Geometry: final body of the model. Coordinates: model frame, mm. Face numbers are marked on the shaded views. A direction names the side the tool comes from. Coordinates: 2 decimals unless noted, no trailing zeros. Order: outer loops, then holes, each group sorted by start corner. A loop starts at its lowest first (then second) coordinate and runs counter-clockwise, first axis right, second up. Notation, with made-up numbers: (81, -4.5) -> (98, -4.5) arc R11 ccw to (98, 1.5) -> close; hole circle Ø11 at (30.5, 37.5). An arc over 180 degrees is marked (long way). Answer in a Markdown table with one row per item. Add a question column.
1) Set-up query: the marked faces 1 and 2. Return all of +Z, -Z, +X, -X, +Y, -Y with unobstructed straight access to the full face (end or side cutting, diameter ignored); none if empty.
2) Contact query for flat-ended pins moving along their axis: P1, Ø1.8, axis at x = -3, z = 17, coming from the +Y side; P2, Ø6, axis at x = -5, y = -48.5, coming from the +Z side; P3, Ø5.5, axis at y = -10.5, z = 29, coming from the -X side. Output: stop coordinate, or through.
3) Ray query, line 1 (Y direction, x = -15.5, z = 19.5); line 2 (X direction, y = -33, z = 18.5); line 3 (X direction, y = -45.5, z = 18.25). Return the intervals inside material, ascending. Write a range as from..to.
4) Section query B-B on z = 20. Return the cut outline in (x, y), then the cut area to 3 significant figures.
5) Section query C-C on y = -20. Return the cut outline in (x, z), then the cut area to 3 significant figures.
```python
from build123d import *

# Parameters (mm, degrees)
F1_DEPTH = 50
F2_W     = 43.9973853057
F2_H     = 6
F3_DEPTH = 125


# Not quite as in the source:
# - ends of sketch curves that miss each other by under 0.0002 mm in the source are joined
# - a feature names something its author has since deleted; it is built from what else it names


with BuildPart() as f1:
    # F0 (on Top) → F1 (new body, symmetric)
    with BuildSketch(Plane.XY):
        Polygon((15.8618143265, -2.6014313847), (15.8618143265, -13.6014313847), (50.9007196128, -13.6014313847), (50.8959237908, -2.6014324301), align=None)
        with BuildLine():
            Line((15.8618143265, -13.6014313847), (-52.0992803872, -13.6014313847))
            ThreePointArc((-52.0992803872, -13.6014313847), (-53.5134939495, -14.1872178223), (-54.0992803872, -15.6014313847))
            Line((-54.0992803872, -15.6014313847), (-54.0992803872, -55.6014313847))
            ThreePointArc((-54.0992803872, -55.6014313847), (-53.5134939495, -57.0156449471), (-52.0992803872, -57.6014313847))
            Line((-52.0992803872, -57.6014313847), (18.8248942664, -57.6014313847))
            ThreePointArc((18.8248942664, -57.6014313847), (20.7365745268, -57.2215481129), (22.3577686464, -56.1396228175))
            Line((22.3577686464, -56.1396228175), (49.4335939928, -29.1044859403))
            ThreePointArc((49.4335939928, -29.1044859403), (50.5193975568, -27.4814483002), (50.9007196128, -25.5662945075))
            Line((50.9007196128, -25.5662945075), (50.9007196128, -13.6014313847))
            Line((50.9007196128, -13.6014313847), (15.8618143265, -13.6014313847))
        make_face()
        with BuildLine():
            ThreePointArc((-30.6326959729, -46.4203889966), (-41.1326959729, -35.9203889966), (-30.6326959729, -25.4203889966))
            Line((-30.6326959729, -25.4203889966), (-9.6326959729, -25.4203889966))
            ThreePointArc((-9.6326959729, -25.4203889966), (0.8673040271, -35.9203889966), (-9.6326959729, -46.4203889966))
            Line((-9.6326959729, -46.4203889966), (-30.6326959729, -46.4203889966))
        make_face(mode=Mode.SUBTRACT)
    extrude(amount=F1_DEPTH, both=True)


with BuildPart() as f3:
    # F2 (on Right) → F3 (new body, symmetric)
    with BuildSketch(Plane.YZ):
        Polygon((-2.610102063, 37.4432504177), (-2.610102063, 31.4432504177), (54.789897937, 31.4432504177), (54.7872818802, 37.4557568013), align=None)
        with BuildLine():
            Line((-8.1155181983, 18.9779470539), (-2.610102063, 31.4432504177))
            Line((-2.610102063, 31.4432504177), (-2.6127167571, 37.443249848))
            ThreePointArc((-2.6127167571, 37.443249848), (-5.8865329423, 36.4696806314), (-8.0986299437, 33.8673093492))
            Line((-8.0986299437, 33.8673093492), (-13.6040460789, 21.4020059854))
            Line((-13.6040460789, 21.4020059854), (-13.6040460789, 15.4020059854))
            ThreePointArc((-13.6040460789, 15.4020059854), (-10.3287104922, 16.3748619856), (-8.1155181983, 18.9779470539))
        make_face()
        Polygon((-2.6127167571, 37.443249848), (-2.610102063, 31.4432504177), (-2.610102063, 37.4432504177), align=None)
        with Locations((-35.6027387318, 18.4020059854)):
            Rectangle(F2_W, F2_H)
    extrude(amount=F3_DEPTH, both=True)

    # F4: intersect F1
    add(f1.part, mode=Mode.INTERSECT)


solid = f3.part
```
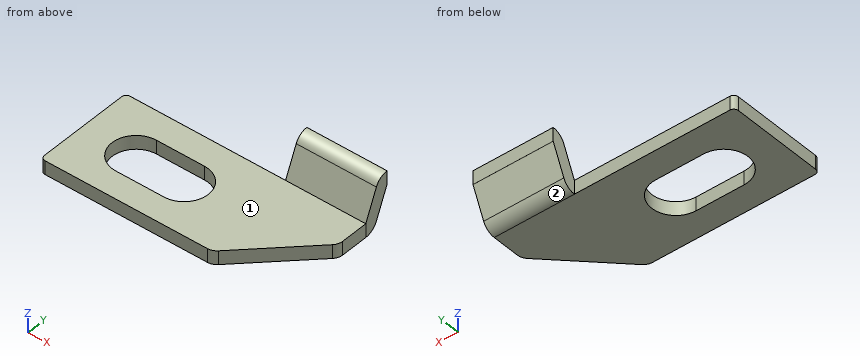
Result:
| question | item | result |
|---|---|---|
| 1 | face 1 | +Z, +X, -X, -Y |
| 1 | face 2 | -Z, +X, -X, +Y |
| 2 | P1 | y = -13.6 |
| 2 | P2 | z = 21.4 |
| 2 | P3 | x = 15.86 |
| 3 | line 1 | -57.6..-46.42, -25.42..-13.6 |
| 3 | line 2 | -54.1..-40.72, 0.45..45.53 |
| 3 | line 3 | -54.1..-34.93, -5.33..33.01 |
| 4 | outline | (-54.1, -55.6) arc R2 ccw to (-52.1, -57.6) -> (18.82, -57.6) arc R5 ccw to (22.36, -56.14) -> (49.43, -29.1) arc R5 ccw to (50.9, -25.57) -> (50.9, -13.6) -> (50.9, -7.66) -> (15.86, -7.66) -> (15.86, -13.6) -> (-52.1, -13.6) arc R2 ccw to (-54.1, -15.6) -> close; hole (-30.63, -46.42) -> (-9.63, -46.42) arc R10.5 ccw to (-9.63, -25.42) -> (-30.63, -25.42) arc R10.5 ccw to start |
| 4 | area | 3,590 mm2 |
| 5 | outline | (-54.1, 15.4) -> (50.9, 15.4) -> (50.9, 21.4) -> (-54.1, 21.4) -> close |
| 5 | area | 630 mm2 |
